For this review, take the finished solid that the model builds, in its own axes (mm). A direction names the side the tool comes from. Coordinates: 2 decimals unless noted, no trailing zeros. Write each loop counter-clockwise with the first axis right and the second up, starting at its lowest first coordinate (ties: lowest second). Pieces come first, ordered by that corner, then holes. Notation, with made-up numbers: (22.25, 27) - (42.25, 27) arc R27 ccw to (42.25, 62) - close; hole circle Ø4 at (51.5, -21). An arc over 180 degrees is marked (long way). Write each question's results on one line, items separated by ' | '.
from build123d import *

# Parameters (mm, degrees)
SKETCH1_R           = 44
BOSS_EXTRUDE1_DEPTH = 14.5
FILLET1_R           = 4
SKETCH2_R           = 18
CUT_EXTRUDE1_DEPTH  = 0.1
SKETCH3_R           = 2.5
CUT_EXTRUDE2_DEPTH  = 64.869867769
SKETCH4_R           = 7.5
SKETCH4_R_2         = 2.5
BOSS_EXTRUDE2_DEPTH = 9.3
CUT_EXTRUDE3_START  = -0.1
SKETCH4_3_R         = 18
SKETCH4_3_R_2       = 7.5
CUT_EXTRUDE3_DEPTH  = 0.1


with BuildPart() as part:
    # Sketch1 → Boss-Extrude1 (new body)
    with BuildSketch(Plane(origin=(0, 0, 0), x_dir=(1, 0, 0), z_dir=(0, 1, 0))):
        with Locations(Location((0, 0, 0), (0, 0, 90))):
            Circle(SKETCH1_R)
    extrude(amount=BOSS_EXTRUDE1_DEPTH)

    # Fillet1
    fillet1_edges = [part.edges().sort_by_distance(p)[0] for p in [
        (0, 14.5, 44),
    ]]
    fillet(fillet1_edges, radius=FILLET1_R)

    # Sketch2 → Cut-Extrude1 (cut)
    with BuildSketch(Plane(origin=(0, 14.5, 0), x_dir=(1, 0, 0), z_dir=(0, 1, 0))):
        with Locations(Location((0, 0, 0), (0, 0, 270))):
            Circle(SKETCH2_R)
    extrude(amount=-CUT_EXTRUDE1_DEPTH, mode=Mode.SUBTRACT)

    # Sketch3 → Cut-Extrude2 (cut, through all)
    with BuildSketch(Plane(origin=(0, 14.4, 0), x_dir=(1, 0, 0), z_dir=(0, 1, 0))):
        with Locations(Location((0, 0, 0), (0, 0, 270))):
            Circle(SKETCH3_R)
    extrude(amount=-CUT_EXTRUDE2_DEPTH, mode=Mode.SUBTRACT)

    # Sketch4 → Boss-Extrude2 (add)
    with BuildSketch(Plane.XZ):
        with Locations(Location((0, 0, 0), (0, 0, 90))):
            Circle(SKETCH4_R)
        with Locations(Location((0, 0, 0), (0, 0, 90))):
            Circle(SKETCH4_R_2, mode=Mode.SUBTRACT)
    extrude(amount=BOSS_EXTRUDE2_DEPTH)

    # Sketch4_3 → Cut-Extrude3 (cut)
    with BuildSketch(Plane.XZ.offset(CUT_EXTRUDE3_START)):
        with Locations(Location((0, 0, 0), (0, 0, 90))):
            Circle(SKETCH4_3_R)
        with Locations(Location((0, 0, 0), (0, 0, 270))):
            Circle(SKETCH4_3_R_2, mode=Mode.SUBTRACT)
    extrude(amount=CUT_EXTRUDE3_DEPTH, mode=Mode.SUBTRACT)


solid = part.part
Q1. For pin 1 (5 mm diameter, centred on x = 27.5, y = 0.5, fed in from +Z); pin 2 (1.5 mm diameter, centred on y = -2, z = 1.5, fed in from +X); pin 3 (11 mm diameter, centred on x = 5, z = 6.5, fed in from +Y), all flat-tipped, find the tip position at first contact; note any pin that passes through.
Results found:
pin 1: z = 36.21 | pin 2: x = 7.46 | pin 3: y = 14.4
Q2. Take a section at D-D on y = -2.25. State the section outline as (x, z) points.
Results found:
outline: circle Ø15 at (0, 0); hole circle Ø5 at (0, 0)
Q3. For faces 4 (the face through (8, 0.1, 0)), 5 (the face through (-2, -9.3, -2)), list the 3-axis set-ups (+Z, -Z, +X, -X, +Y, -Y) from which the entire face can be reached by the end or side of a thin tool; tool diameter is ignored.
Results found:
face 4: -Y | face 5: +Z, -Z, +X, -X, -Y
Q4. Mouldability with a two-part tool opening along Z and no side actions: class faces 1 (the face through (8, 14.5, -17)), 2 (the face through (42.954, 5.176, 9.538)), 3 (the face through (-4, 14.4, 0)) as pulls with the +Z half, pulls with the -Z half, needs draft (parallel to the pull), parting line crosses it, or undercut.
Results found:
face 1: needs draft | face 2: parting line crosses it | face 3: undercut
Q5. Take a section at B-B on x = 0. State the section outline as (y, z) points.
Results found:
outline: (-9.3, -7.5) - (0.1, -7.5) - (0.1, -18) - (0, -18) - (0, -44) - (10.5, -44) arc R4 ccw to (14.5, -40) - (14.5, -18) - (14.4, -18) - (14.4, -2.5) - (-9.3, -2.5) - close; (-9.3, 2.5) - (14.4, 2.5) - (14.4, 18) - (14.5, 18) - (14.5, 40) arc R4 ccw to (10.5, 44) - (0, 44) - (0, 18) - (0.1, 18) - (0.1, 7.5) - (-9.3, 7.5) - close
Q6. Take a section at C-C on y = 5. State the section outline as (x, z) points, plus the area to 3 significant figures.
Results found:
outline: circle Ø88 at (0, 0); hole circle Ø5 at (0, 0) | area: 6,060 mm2
Q7. Wall thickness on line 1 along X through (y, z) = (2.5, 0); line 2 along X through (y, z) = (-0.5, 0); line 3 along Y through (x, z) = (-3.5, 26): over which ranges is each line inside the solid? List them lowest first. Write a range as from..to.
Results found:
line 1: -44..-2.5, 2.5..44 | line 2: -7.5..-2.5, 2.5..7.5 | line 3: 0..14.5
Q8. Take a section at A-A on z = 0. State the section outline as (x, y) points, plus the area to 3 significant figures.
Results found:
outline: (-44, 0) - (-18, 0) - (-18, 0.1) - (-7.5, 0.1) - (-7.5, -9.3) - (-2.5, -9.3) - (-2.5, 14.4) - (-18, 14.4) - (-18, 14.5) - (-40, 14.5) arc R4 ccw to (-44, 10.5) - close; (2.5, -9.3) - (7.5, -9.3) - (7.5, 0.1) - (18, 0.1) - (18, 0) - (44, 0) - (44, 10.5) arc R4 ccw to (40, 14.5) - (18, 14.5) - (18, 14.4) - (2.5, 14.4) - close | area: 1,280 mm2
